Geometry check sheet. Reference: the model listing, model coordinates, mm. Face numbers are marked on the shaded views. A direction names the side the tool comes from. Give positions to 0.01 mm unless a question says otherwise; leave off trailing zeros. Write each loop counter-clockwise with the first axis right and the second up, starting at its lowest first coordinate (ties: lowest second). Pieces come first, ordered by that corner, then holes. Notation, with made-up numbers: (72.25, -6.5) - (107.25, -6.5) arc R27 cw to (107.25, 22.5) - close; hole circle Ø4 at (-10.75, -35.75). An arc over 180 degrees is marked (long way). Use a Markdown table: item, result.
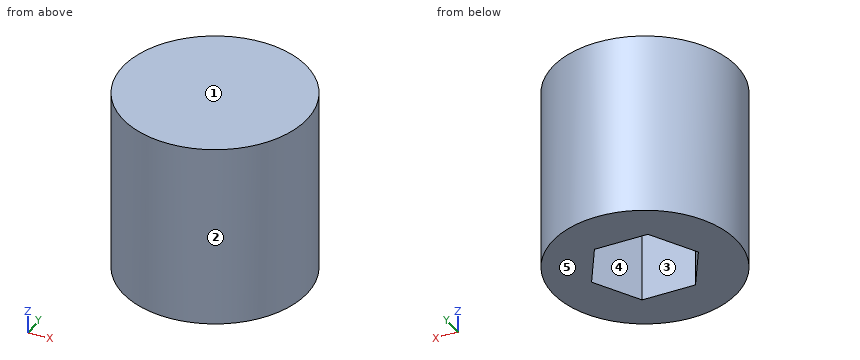
Autodesk Inventor part; units mm, degrees
ref_plane "YZ Plane" through (0, 0, 0) normal (1, 0, 0) x (0, 1, 0)
ref_plane "XZ Plane" through (0, 0, 0) normal (0, 1, 0) x (-1, 0, 0)
ref_plane "XY Plane" through (0, 0, 0) normal (0, 0, 1) x (1, 0, 0)
sketch "Sketch1" plane through (0, 0, 0) normal (0, 0, 1) x (1, 0, 0)
  circle A0 centre (0, 0) radius 5
  dimension "d0" = 10
extrude "Extrusion1" add sketch "Sketch1" along normal blind 10
thread "Thread1"
sketch "Sketch2" plane through (0, 0, 0) normal (0, 0, -1) x (-1, 0, 0)
  circle A0 centre (0, 0) radius 5
  circle A1 centre (0, 0) radius 2.5
  line L0 (-1.8795, -2.5) -> (1.9053, -2.5)
  line L1 (1.2253, -2.8777) -> (3.1177, 0.4)
  line L2 (3.1048, -0.3777) -> (1.2124, 2.9)
  line L3 (1.8795, 2.5) -> (-1.9053, 2.5)
  line L4 (-1.2253, 2.8777) -> (-3.1177, -0.4)
  line L5 (-3.1048, 0.3777) -> (-1.2124, -2.9)
  line L6 (-1.4434, 2.5) -> (1.4434, 2.5)
  line L7 (1.4434, 2.5) -> (2.8868, 0)
  line L8 (2.8868, 0) -> (1.4434, -2.5)
  line L9 (1.4434, -2.5) -> (-1.4434, -2.5)
  line L10 (-1.4434, -2.5) -> (-2.8868, 0)
  line L11 (-2.8868, 0) -> (-1.4434, 2.5)
  dimension "d5" = 5
  dimension "d8" = 360
extrude "Extrusion2" cut sketch "Sketch2" against normal blind 5 contours A1 | A1 L2 L1 | A1 L3 L2 | L1 L0 A1 | A1 L4 L3 | L0 L5 A1 | A1 L5 L4
properties part number "Pusher.Socketscrew"
1) Section check B-B on z = 4.5. Record the boundary of the cut face in (x, y), then the cut area to 3 significant figures.
Working result:
| item | result |
|---|---|
| outline | circle Ø10 at (0, 0); hole (-2.89, 0) - (-1.44, -2.5) - (1.44, -2.5) - (2.89, 0) - (1.44, 2.5) - (-1.44, 2.5) - close |
| area | 56.9 mm² |
2) Mould release check, pull along Y, two halves, no side actions. Record for the marked faces 1, 2 and 3: pulls with the +Y half, pulls with the -Y half, needs draft (parallel to the pull), parting line crosses it, or undercut.
Working result:
| item | result |
|---|---|
| face 1 | needs draft |
| face 2 | parting line crosses it |
| face 3 | undercut |
3) Set-up check for the marked faces 4 and 5: record each of +Z, -Z, +X, -X, +Y, -Y from which the full face is reachable in a straight line by a thin tool's end or side.
Working result:
| item | result |
|---|---|
| face 4 | -Z |
| face 5 | -Z, +X, -X, +Y, -Y |
4) Depth check by flat-ended pin: P1, Ø2, axis at y = 4, z = 4, coming from the +X side; P2, Ø1.5, axis at x = 1.5, y = 0.5, coming from the -Z side; P3, Ø2, axis at x = -1.5, y = -3, coming from the -Z side. Enter the tip coordinate at first touch or a pass-through.
Working result:
| item | result |
|---|---|
| P1 | stops at x = 4 |
| P2 | stops at z = 5 |
| P3 | stops at z = 0 |
5) Section check C-C on y = -2. Record the boundary of the cut face in (x, z), then the cut area to 3 significant figures.
Working result:
| item | result |
|---|---|
| outline | (-4.58, 0) - (-1.73, 0) - (-1.73, 5) - (1.73, 5) - (1.73, 0) - (4.58, 0) - (4.58, 10) - (-4.58, 10) - close |
| area | 74.3 mm² |
6) Section check A-A on x = 0. Record the boundary of the cut face in (y, z), then the cut area to 3 significant figures.
Working result:
| item | result |
|---|---|
| outline | (-5, 0) - (-2.5, 0) - (-2.5, 5) - (2.5, 5) - (2.5, 0) - (5, 0) - (5, 10) - (-5, 10) - close |
| area | 75.0 mm² |
7) Material ranges on L1, parallel to Y at x = 0, z = 4.5; L2, parallel to Y at x = 1.75, z = 1.25; L3, parallel to X at y = 1, z = 1, recorded low to high. Write a range as from..to.
Working result:
| item | result |
|---|---|
| L1 | y = -5..-2.5, 2.5..5 |
| L2 | y = -4.68..-1.97, 1.97..4.68 |
| L3 | x = -4.9..-2.31, 2.31..4.9 |
8) Section check D-D on z = 8.25. Record the boundary of the cut face in (x, y), then the cut area to 3 significant figures.
Working result:
| item | result |
|---|---|
| outline | circle Ø10 at (0, 0) |
| area | 78.5 mm² |
